Read the model definition and answer for the solid it produces. Units are mm, in the model's axes. A direction names the side the tool comes from. Coordinates: 2 decimals unless noted, no trailing zeros. Write each loop counter-clockwise with the first axis right and the second up, starting at its lowest first coordinate (ties: lowest second). Pieces come first, ordered by that corner, then holes. Notation, with made-up numbers: (68.25, 1) -> (108.25, 1) arc R20 ccw to (108.25, 9) -> close; hole circle Ø5 at (87, 11.5). An arc over 180 degrees is marked (long way). Answer as a JSON object with one key per item and string values. Group by question number.
(1) Flat-ended cylindrical pins translate along their axes: P1, Ø16, axis at x = 45.99, y = 11.28, coming from the -Z side; P2, Ø9, axis at x = 45, y = 13, coming from the +Z side. Find the tip coordinate at first contact, or state that the pin passes through.
(2) For a pull along Y with two mould halves and no side action, classify faces 4 (the face through (-1, -49.677, 38)), 5 (the face through (-12.772, 24.225, 34.436)), 6 (the face through (15, -11, 0)) as +Y half, -Y half, draft (parallel to the pull), parting line (faces both ways), or undercut.
(3) Straight lines are drawn through the part: L1, parallel to Y at x = 29, z = 10.5; L2, parallel to X at y = 23, z = 34; L3, parallel to Z at x = -69, y = 23. For each, find the intervals that lie inside material, in ascending order.
(4) Find section A-A (x = -65). Give the vertices of the cut face in (y, z).
(5) Which of the six approach directions +Z, -Z, +X, -X, +Y, -Y give full straight-line access (tool end or side, diameter ignored) to faces 1 (the face through (-15, 11, 2.5)), 2 (the face through (-46, 34, 0)), 3 (the face through (-1, -45.72, 34))?
(6) Find section B-B (z = 51.5). Count the separate pieces of the cut face and the enclosed holes in it, then the cut area to 3 significant figures.
from build123d import *

# Parameters (mm, degrees)
F0_W     = 152.4
F0_H     = 101.6
F0_R     = 8.89
F1_DEPTH = 2.5
F2_DEPTH = 76.2
F4_W     = 142.24
F4_H     = 91.44
F4_R     = 10.16
F5_DEPTH = 69.85


with BuildPart() as f1:
    # F0 (on Top) → F1 (new body)
    with BuildSketch(Plane.XY):
        with Locations((0.2656728029, 1.1231710495)):
            Rectangle(F0_W, F0_H)
        with Locations((-45.4543271971, -34.4368289505)):
            Circle(F0_R, mode=Mode.SUBTRACT)
        with Locations((-14.9743271971, -34.4368289505)):
            Circle(F0_R, mode=Mode.SUBTRACT)
        with Locations((-45.4543271971, -11.5768289505)):
            Circle(F0_R, mode=Mode.SUBTRACT)
        with Locations((-14.9743271971, -11.5768289505)):
            Circle(F0_R, mode=Mode.SUBTRACT)
        with Locations((15.5056728029, -34.4368289505)):
            Circle(F0_R, mode=Mode.SUBTRACT)
        with Locations((45.9856728029, -34.4368289505)):
            Circle(F0_R, mode=Mode.SUBTRACT)
        with Locations((15.5056728029, -11.5768289505)):
            Circle(F0_R, mode=Mode.SUBTRACT)
        with Locations((45.9856728029, -11.5768289505)):
            Circle(F0_R, mode=Mode.SUBTRACT)
        with Locations((-45.4543271971, 11.2831710495)):
            Circle(F0_R, mode=Mode.SUBTRACT)
        with Locations((-14.9743271971, 11.2831710495)):
            Circle(F0_R, mode=Mode.SUBTRACT)
        with Locations((-45.4543271971, 34.1431710495)):
            Circle(F0_R, mode=Mode.SUBTRACT)
        with Locations((-14.9743271971, 34.1431710495)):
            Circle(F0_R, mode=Mode.SUBTRACT)
        with Locations((15.5056728029, 11.2831710495)):
            Circle(F0_R, mode=Mode.SUBTRACT)
        with Locations((45.9856728029, 11.2831710495)):
            Circle(F0_R, mode=Mode.SUBTRACT)
        with Locations((15.5056728029, 34.1431710495)):
            Circle(F0_R, mode=Mode.SUBTRACT)
        with Locations((45.9856728029, 34.1431710495)):
            Circle(F0_R, mode=Mode.SUBTRACT)
        with Locations((-45.4543271971, -34.4368289505)):
            Circle(F0_R)
        with Locations((-14.9743271971, -34.4368289505)):
            Circle(F0_R)
        with Locations((-14.9743271971, -11.5768289505)):
            Circle(F0_R)
        with Locations((-45.4543271971, -11.5768289505)):
            Circle(F0_R)
        with Locations((-45.4543271971, 11.2831710495)):
            Circle(F0_R)
        with Locations((-45.4543271971, 34.1431710495)):
            Circle(F0_R)
        with Locations((-14.9743271971, 34.1431710495)):
            Circle(F0_R)
        with Locations((-14.9743271971, 11.2831710495)):
            Circle(F0_R)
        with Locations((15.5056728029, 34.1431710495)):
            Circle(F0_R)
        with Locations((15.5056728029, 11.2831710495)):
            Circle(F0_R)
        with Locations((15.5056728029, -11.5768289505)):
            Circle(F0_R)
        with Locations((15.5056728029, -34.4368289505)):
            Circle(F0_R)
        with Locations((45.9856728029, -34.4368289505)):
            Circle(F0_R)
        with Locations((45.9856728029, -11.5768289505)):
            Circle(F0_R)
        with Locations((45.9856728029, 11.2831710495)):
            Circle(F0_R)
        with Locations((45.9856728029, 34.1431710495)):
            Circle(F0_R)
    extrude(amount=F1_DEPTH)

    # F0 (on Top) → F2 (join)
    with BuildSketch(Plane.XY):
        with Locations((0.2656728029, 1.1231710495)):
            Rectangle(F0_W, F0_H)
        with Locations((-45.4543271971, -34.4368289505)):
            Circle(F0_R, mode=Mode.SUBTRACT)
        with Locations((-14.9743271971, -34.4368289505)):
            Circle(F0_R, mode=Mode.SUBTRACT)
        with Locations((-45.4543271971, -11.5768289505)):
            Circle(F0_R, mode=Mode.SUBTRACT)
        with Locations((-14.9743271971, -11.5768289505)):
            Circle(F0_R, mode=Mode.SUBTRACT)
        with Locations((15.5056728029, -34.4368289505)):
            Circle(F0_R, mode=Mode.SUBTRACT)
        with Locations((45.9856728029, -34.4368289505)):
            Circle(F0_R, mode=Mode.SUBTRACT)
        with Locations((15.5056728029, -11.5768289505)):
            Circle(F0_R, mode=Mode.SUBTRACT)
        with Locations((45.9856728029, -11.5768289505)):
            Circle(F0_R, mode=Mode.SUBTRACT)
        with Locations((-45.4543271971, 11.2831710495)):
            Circle(F0_R, mode=Mode.SUBTRACT)
        with Locations((-14.9743271971, 11.2831710495)):
            Circle(F0_R, mode=Mode.SUBTRACT)
        with Locations((-45.4543271971, 34.1431710495)):
            Circle(F0_R, mode=Mode.SUBTRACT)
        with Locations((-14.9743271971, 34.1431710495)):
            Circle(F0_R, mode=Mode.SUBTRACT)
        with Locations((15.5056728029, 11.2831710495)):
            Circle(F0_R, mode=Mode.SUBTRACT)
        with Locations((45.9856728029, 11.2831710495)):
            Circle(F0_R, mode=Mode.SUBTRACT)
        with Locations((15.5056728029, 34.1431710495)):
            Circle(F0_R, mode=Mode.SUBTRACT)
        with Locations((45.9856728029, 34.1431710495)):
            Circle(F0_R, mode=Mode.SUBTRACT)
    extrude(amount=F2_DEPTH)

    # F4 (on face) → F5 (cut)
    with BuildSketch(Plane.XY):
        Rectangle(F4_W, F4_H)
        with Locations((-45.4543271971, -34.4368289505)):
            Circle(F4_R, mode=Mode.SUBTRACT)
        with Locations((-14.9743271971, -34.4368289505)):
            Circle(F4_R, mode=Mode.SUBTRACT)
        with Locations((-45.4543271971, -11.5768289505)):
            Circle(F4_R, mode=Mode.SUBTRACT)
        with Locations((-14.9743271971, -11.5768289505)):
            Circle(F4_R, mode=Mode.SUBTRACT)
        with Locations((15.5056728029, -34.4368289505)):
            Circle(F4_R, mode=Mode.SUBTRACT)
        with Locations((45.9856728029, -34.4368289505)):
            Circle(F4_R, mode=Mode.SUBTRACT)
        with Locations((15.5056728029, -11.5768289505)):
            Circle(F4_R, mode=Mode.SUBTRACT)
        with Locations((45.9856728029, -11.5768289505)):
            Circle(F4_R, mode=Mode.SUBTRACT)
        with Locations((-45.4543271971, 11.2831710495)):
            Circle(F4_R, mode=Mode.SUBTRACT)
        with Locations((-14.9743271971, 11.2831710495)):
            Circle(F4_R, mode=Mode.SUBTRACT)
        with Locations((-45.4543271971, 34.1431710495)):
            Circle(F4_R, mode=Mode.SUBTRACT)
        with BuildLine():
            ThreePointArc((-4.8143271971, 34.1431710495), (-14.9743271971, 23.9831710495), (-25.1343271971, 34.1431710495))
            ThreePointArc((-25.1343271971, 34.1431710495), (-14.9743271971, 44.3031710495), (-4.8143271971, 34.1431710495))
        make_face(mode=Mode.SUBTRACT)
        with Locations((15.5056728029, 11.2831710495)):
            Circle(F4_R, mode=Mode.SUBTRACT)
        with Locations((45.9856728029, 11.2831710495)):
            Circle(F4_R, mode=Mode.SUBTRACT)
        with Locations((15.5056728029, 34.1431710495)):
            Circle(F4_R, mode=Mode.SUBTRACT)
        with Locations((45.9856728029, 34.1431710495)):
            Circle(F4_R, mode=Mode.SUBTRACT)
    extrude(amount=F5_DEPTH, mode=Mode.SUBTRACT)


solid = f1.part
Results below:
{
 "1": {"P1": "stops at z = 0", "P2": "stops at z = 2.5"},
 "2": {"face 4": "-Y half", "face 5": "undercut", "face 6": "draft"},
 "3": {"L1": "y = -49.68 to -45.72, 45.72 to 51.92", "L2": "x = -75.93 to -71.12, 71.12 to 76.47", "L3": "z = 69.85 to 76.2"},
 "4": {"outline": "(-49.68, 0) -> (-45.72, 0) -> (-45.72, 69.85) -> (45.72, 69.85) -> (45.72, 0) -> (51.92, 0) -> (51.92, 76.2) -> (-49.68, 76.2) -> close"},
 "5": {"face 1": "+Z", "face 2": "-Z, +X, -X, +Y, -Y", "face 3": "-Z"},
 "6": {"separate pieces": "17", "enclosed holes": "17", "area": "3,690 mm2"}
}
